CAD build for the part. Positions are in the model's coordinates, mm. A direction names the side the tool comes from. Give positions to 0.01 mm unless a question says otherwise; leave off trailing zeros. Write each loop counter-clockwise with the first axis right and the second up, starting at its lowest first coordinate (ties: lowest second). Pieces come first, ordered by that corner, then holes. Notation, with made-up numbers: (-36.5, 58) - (4.5, 58) arc R24 ccw to (4.5, 72) - close; hole circle Ø3 at (-35.75, -36). An arc over 180 degrees is marked (long way). Answer as a JSON object with one key per item and string values.
from build123d import *

# Parameters (mm, degrees)
SKETCH003_W     = 1.5
SKETCH003_H     = 10.5
SKETCH_R        = 6
SKETCH_R_2      = 1.6
PAD_DEPTH       = 15
SKETCH001_R     = 3.2
POCKET_DEPTH    = 8
SKETCH002_R     = 6
SKETCH002_R_2   = 4
POCKET001_DEPTH = 2


with BuildPart() as revolution:
    # Sketch003 → Revolution (revolve)
    with BuildSketch(Plane.XZ):
        with Locations((5.25, 8.75)):
            Rectangle(SKETCH003_W, SKETCH003_H)
    revolve(axis=Axis((0, 0, 0), (0, 0, 1)))


with BuildPart() as cut:
    # Sketch → Pad (new body)
    with BuildSketch(Plane.XY):
        Circle(SKETCH_R)
        Circle(SKETCH_R_2, mode=Mode.SUBTRACT)
    extrude(amount=PAD_DEPTH)

    # Sketch001 → Pocket (cut)
    with BuildSketch(Plane.XY.offset(15)):
        Circle(SKETCH001_R)
    extrude(amount=-POCKET_DEPTH, mode=Mode.SUBTRACT)

    # Sketch002 → Pocket001 (cut)
    with BuildSketch(Plane(origin=(0, 0, 0), x_dir=(1, 0, 0), z_dir=(0, 0, -1))):
        Circle(SKETCH002_R)
        Circle(SKETCH002_R_2, mode=Mode.SUBTRACT)
    extrude(amount=-POCKET001_DEPTH, mode=Mode.SUBTRACT)

    # Cut: cut Revolution
    add(revolution.part, mode=Mode.SUBTRACT)


solid = cut.part
Item 1: Which spindle directions (+Z, -Z, +X, -X, +Y, -Y) get a long thin tool onto all of the face, cutting with end or side? Do faces 5 (the flat face through (1.4, -1.4, 7)), 6 (the flat face through (1.4, 4.5, 3.5)), 7 (the cylindrical face through (-0.867, 3.905, 0.986)). Say none if no direction does.
Entries:
{"face 5": "+Z", "face 6": "none", "face 7": "-Z"}
Item 2: Probe line 1 (Z direction, x = 0.25, y = 5.25); line 2 (Y direction, x = 0, z = 1.5); line 3 (X direction, y = 0, z = 2.75). List the from-to ranges inside material, lowest first. Write a range as from..to.
Entries:
{"line 1": "2..3.5, 14..15", "line 2": "-4..-1.6, 1.6..4", "line 3": "-6..-1.6, 1.6..6"}
Item 3: Cut at D-D (y = 3.5). Give the cut face in (x, z), and give its area (3 significant figures).
Entries:
{"outline": "(-4.87, 2) - (-1.94, 2) - (-1.94, 0) - (1.94, 0) - (1.94, 2) - (4.87, 2) - (4.87, 3.5) - (2.83, 3.5) - (2.83, 14) - (4.87, 14) - (4.87, 15) - (-4.87, 15) - (-4.87, 14) - (-2.83, 14) - (-2.83, 3.5) - (-4.87, 3.5) - close", "area": "91.5 mm2"}
Item 4: Flat gauge pins, fed straight in: P1, Ø1.5, axis at x = 4, z = 8, coming from the +Y side; P2, Ø2, axis at x = 1, y = 1, coming from the +Z side; P3, Ø3, axis at y = -4, z = 11, coming from the -X side. Where does each tip first touch, or does it go through?
Entries:
{"P1": "y = 3.11", "P2": "z = 7", "P3": "x = -3.74"}
Item 5: Mould opens along X. For faces 1 (the flat face through (2, 0, 0)), 2 (the cylindrical face through (-1.27, -0.97, 3.45)), 3 (the cylindrical face through (-2.539, -1.947, 11.056)), 4 (the cylindrical face through (-6, 0, 3)) say: +X half, -X half, draft (parallel to the pull), parting line (faces both ways), or undercut.
Entries:
{"face 1": "draft", "face 2": "undercut", "face 3": "undercut", "face 4": "parting line"}
Item 6: Cut at C-C (z = 3.75). Give the cut face in (x, y).
Entries:
{"outline": "circle Ø9 at (0, 0); hole circle Ø3.2 at (0, 0)"}
Item 7: Cut at A-A (x = 0). Give the cut face in (y, z).
Entries:
{"outline": "(-6, 2) - (-4, 2) - (-4, 0) - (-1.6, 0) - (-1.6, 7) - (-3.2, 7) - (-3.2, 15) - (-6, 15) - (-6, 14) - (-4.5, 14) - (-4.5, 3.5) - (-6, 3.5) - close; (1.6, 0) - (4, 0) - (4, 2) - (6, 2) - (6, 3.5) - (4.5, 3.5) - (4.5, 14) - (6, 14) - (6, 15) - (3.2, 15) - (3.2, 7) - (1.6, 7) - close"}
